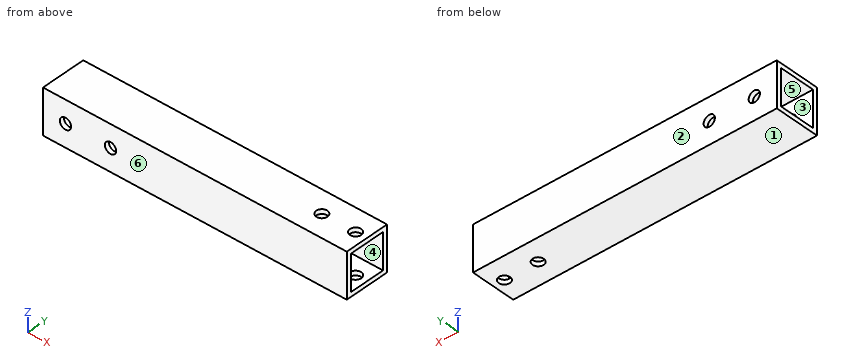
from build123d import *

# Parameters (mm, degrees)
SKETCH1_W           = 20
SKETCH1_H           = 20
SKETCH1_W_2         = 16
SKETCH1_H_2         = 16
BOSS_EXTRUDE1_DEPTH = 135
SKETCH2_R           = 2.5
CUT_EXTRUDE1_DEPTH  = 137.839321834
SKETCH3_R           = 2.5
CUT_EXTRUDE2_DEPTH  = 137.839321834


with BuildPart() as part:
    # Sketch1 → Boss-Extrude1 (new body)
    with BuildSketch(Plane(origin=(0, 0, 0), x_dir=(0, 0, -1), z_dir=(1, 0, 0))):
        Rectangle(SKETCH1_W, SKETCH1_H)
        Rectangle(SKETCH1_W_2, SKETCH1_H_2, mode=Mode.SUBTRACT)
    extrude(amount=BOSS_EXTRUDE1_DEPTH)

    # Sketch2 → Cut-Extrude1 (cut, through all)
    with BuildSketch(Plane.XY.offset(10)):
        with Locations((130, 0)):
            Circle(SKETCH2_R)
        with Locations((115, 0)):
            Circle(SKETCH2_R)
    extrude(amount=-CUT_EXTRUDE1_DEPTH, mode=Mode.SUBTRACT)

    # Sketch3 → Cut-Extrude2 (cut, through all)
    with BuildSketch(Plane(origin=(0, 10, 0), x_dir=(1, 0, 0), z_dir=(0, 1, 0))):
        with Locations(Location((10, 0, 0), (0, 0, 270))):
            Circle(SKETCH3_R)
        with Locations(Location((30, 0, 0), (0, 0, 270))):
            Circle(SKETCH3_R)
    extrude(amount=-CUT_EXTRUDE2_DEPTH, mode=Mode.SUBTRACT)


solid = part.part
The listing builds one solid part. Answer for the finished solid, in the listing's coordinates (mm). Face numbers are marked on the shaded views. A direction names the side the tool comes from. Give positions to 0.01 mm unless a question says otherwise; leave off trailing zeros. Write each loop counter-clockwise with the first axis right and the second up, starting at its lowest first coordinate (ties: lowest second). Pieces come first, ordered by that corner, then holes. Notation, with made-up numbers: (51, 30.25) - (77, 30.25) arc R11 cw to (77, 41.25) - close; hole circle Ø1 at (28.5, -18). An arc over 180 degrees is marked (long way). Use a Markdown table: item, result.
1. Find the intervals of material crossed by probe 1 along X at (y, z) = (-8.6, 0); probe 2 along Z at (x, y) = (25.5, 3.5), in increasing order. Write a range as from..to.
Values follow:
| item | result |
|---|---|
| probe 1 | x = 0..7.5, 12.5..27.5, 32.5..135 |
| probe 2 | z = -10..-8, 8..10 |
2. A tool of negligible diameter and unlimited length cuts with its end or side. For the marked faces 5 and 6, from which of +Z, -Z, +X, -X, +Y, -Y can it reach the whole face along a straight path? Write none if from no direction.
Values follow:
| item | result |
|---|---|
| face 5 | +X, -X |
| face 6 | +Z, -Z, +X, -X, -Y |
3. Section B-B on y = 4.75 is taken. Write down the section's boundary in (x, z), plus the area to 3 significant figures.
Values follow:
| item | result |
|---|---|
| outline | (0, -10) - (135, -10) - (135, -8) - (0, -8) - close; (0, 8) - (135, 8) - (135, 10) - (0, 10) - close |
| area | 540 mm² |
4. For a pull along Y with two mould halves and no side action, classify the marked faces 1, 2, 3 and 4 as released by +Y, released by -Y, zero draft, split by the parting line, or undercut.
Values follow:
| item | result |
|---|---|
| face 1 | zero draft |
| face 2 | released by +Y |
| face 3 | undercut |
| face 4 | undercut |
5. Each of these flat-tipped pins is pushed along its axis until it touches: P1, Ø10, axis at y = -2.5, z = -4, coming from the -X side; P2, Ø4, axis at x = 30, z = 0, coming from the +Y side. Where does it stop, or does it pass through?
Values follow:
| item | result |
|---|---|
| P1 | stops at x = 0 |
| P2 | passes through |
6. Section D-D on x = 79 is taken. Write down the section's boundary in (y, z), plus the area to 3 significant figures.
Values follow:
| item | result |
|---|---|
| outline | (-10, -10) - (10, -10) - (10, 10) - (-10, 10) - close; hole (-8, -8) - (8, -8) - (8, 8) - (-8, 8) - close |
| area | 144 mm² |
7. Section C-C on z = 0 is taken. Write down the section's boundary in (x, y).
Values follow:
| item | result |
|---|---|
| outline | (0, -10) - (7.5, -10) - (7.5, -8) - (0, -8) - close; (0, 8) - (7.5, 8) - (7.5, 10) - (0, 10) - close; (12.5, -10) - (27.5, -10) - (27.5, -8) - (12.5, -8) - close; (12.5, 8) - (27.5, 8) - (27.5, 10) - (12.5, 10) - close; (32.5, -10) - (135, -10) - (135, -8) - (32.5, -8) - close; (32.5, 8) - (135, 8) - (135, 10) - (32.5, 10) - close |
8. Section A-A on x = 10 is taken. Write down the section's boundary in (y, z), plus the area to 3 significant figures.
Values follow:
| item | result |
|---|---|
| outline | (-10, -10) - (10, -10) - (10, -2.5) - (8, -2.5) - (8, -8) - (-8, -8) - (-8, -2.5) - (-10, -2.5) - close; (-10, 2.5) - (-8, 2.5) - (-8, 8) - (8, 8) - (8, 2.5) - (10, 2.5) - (10, 10) - (-10, 10) - close |
| area | 124 mm² |
